Could you check a few things on this drawing? It's one solid part, dimensions in mm from its lowest x, y, z. Round coordinates to 2 decimals unless told otherwise and drop trailing zeros. Write each loop counter-clockwise with the first axis right and the second up, starting at its lowest first coordinate (ties: lowest second). Pieces come first, ordered by that corner, then holes. Notation, with made-up numbers: (75.25, -24.5) -> (92.25, -24.5) arc R26 cw to (92.25, 11.5) -> close; hole circle Ø11 at (-13, -10.75). An arc over 180 degrees is marked (long way). Answer in a Markdown table with one row per item.
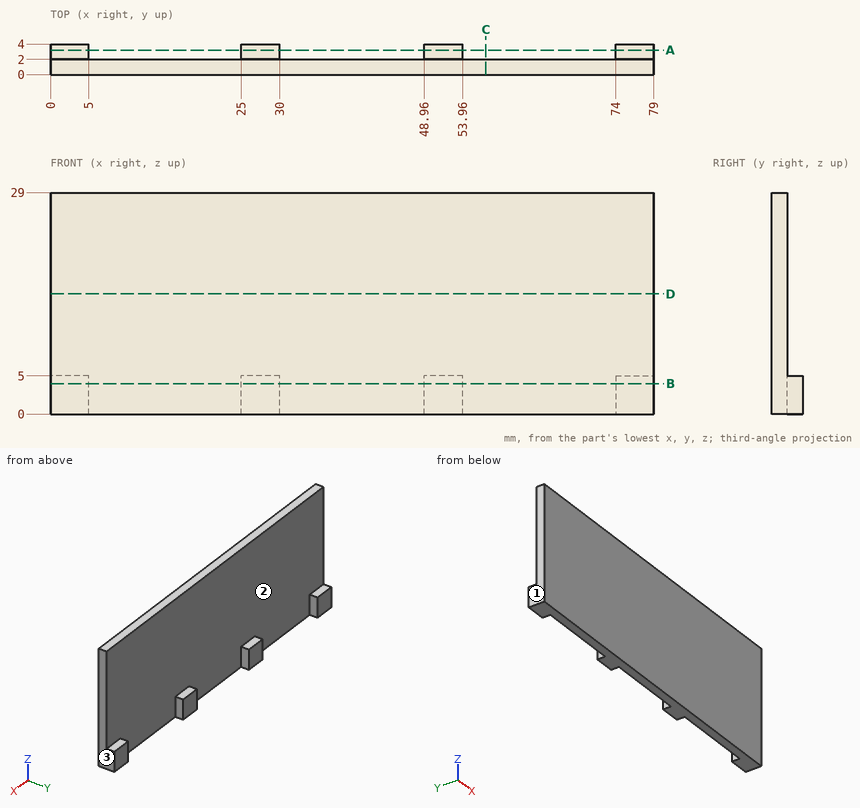
1) Imagine slicing it at A-A, the plane y = 3.2. Please give me the cut outline in (x, z).
Findings:
| item | result |
|---|---|
| outline | (0, 0) -> (5, 0) -> (5, 5) -> (0, 5) -> close; (25, 0) -> (30, 0) -> (30, 5) -> (25, 5) -> close; (48.96, 0) -> (53.96, 0) -> (53.96, 5) -> (48.96, 5) -> close; (74, 0) -> (79, 0) -> (79, 5) -> (74, 5) -> close |
2) Imagine slicing it at B-B, the plane z = 4. Please give me the cut outline in (x, y).
Findings:
| item | result |
|---|---|
| outline | (0, 0) -> (79, 0) -> (79, 4) -> (74, 4) -> (74, 2) -> (53.96, 2) -> (53.96, 4) -> (48.96, 4) -> (48.96, 2) -> (30, 2) -> (30, 4) -> (25, 4) -> (25, 2) -> (5, 2) -> (5, 4) -> (0, 4) -> close |
3) Thinking about a two-plate mould opening in X: for the marked faces 1, 2 and 3, which applies, +X half, -X half, draft (parallel to the pull), parting line (faces both ways), or undercut?
Findings:
| item | result |
|---|---|
| face 1 | -X half |
| face 2 | undercut |
| face 3 | +X half |
4) Imagine slicing it at D-D, the plane z = 15.75. Please give me the cut outline in (x, y), plus the area to 3 significant figures.
Findings:
| item | result |
|---|---|
| outline | (0, 0) -> (79, 0) -> (79, 2) -> (0, 2) -> close |
| area | 158 mm^2 |
5) Imagine slicing it at C-C, the plane x = 57. Please give me the cut outline in (y, z), plus the area to 3 significant figures.
Findings:
| item | result |
|---|---|
| outline | (0, 0) -> (2, 0) -> (2, 29) -> (0, 29) -> close |
| area | 58.0 mm^2 |
6) For pin 1 (1 mm diameter, centred on x = 1.5, y = 3.5, fed in from +Z); pin 2 (1 mm diameter, centred on x = 44, z = 23, fed in from +Y), each with a flat end and sliding along its axis, tell me the tip position at first contact or that it passes through.
Findings:
| item | result |
|---|---|
| pin 1 | stops at z = 5 |
| pin 2 | stops at y = 2 |
7) Please list where this line runs through material, in increasing order: line 1 (Y direction, x = 12, z = 5.5).
Findings:
| item | result |
|---|---|
| line 1 | y = 0 to 2 |
